from build123d import *

# Parameters (mm, degrees)
EXTRUDE_1_DEPTH        = 3
SKETCH_2_R             = 1.5
SKETCH_2_R_2           = 13.5
CUT_EXTRUDE_1333_DEPTH = 144.209636547
SKETCH_3_OUTSIDE_W     = 225.27
SKETCH_3_OUTSIDE_H     = 165.27
CUT_EXTRUDE_1_DEPTH    = 144.209636547
SKETCH_5_R             = 1.5
SKETCH_5_R_2           = 2
CUT_EXTRUDE_3_DEPTH    = 121.819741764
SKETCH_4_W             = 7
SKETCH_4_H             = 16
CUT_EXTRUDE_2_DEPTH    = 121.819741764
FILLET_1_R             = 2


with BuildPart() as part:
    # 草图1 → 凸台-拉伸1 (new body)
    with BuildSketch(Plane(origin=(0, 0, 0), x_dir=(1, 0, 0), z_dir=(0, 1, 0))):
        Polygon((-30, 60), (30, 60), (30, 33), (130, 33), (130, -33), (30, -33), (30, -60), (-30, -60), (-30, -30), (-50, -30), (-50, 30), (-30, 30), align=None)
    extrude(amount=EXTRUDE_1_DEPTH)

    # 草图2 → Cut-Extrude 1333 (cut, through all)
    with BuildSketch(Plane(origin=(0, 3, 0), x_dir=(1, 0, 0), z_dir=(0, 1, 0))):
        with Locations(Location((-30, 13, 0), (0, 0, 270))):
            Circle(SKETCH_2_R)
        with Locations(Location((-30, -13, 0), (0, 0, 270))):
            Circle(SKETCH_2_R)
        with Locations(Location((17.5, 36.9, 0), (0, 0, 270))):
            Circle(SKETCH_2_R)
        with Locations(Location((12.374368671, 24.525631329, 0), (0, 0, 270))):
            Circle(SKETCH_2_R)
        with Locations(Location((0, 19.4, 0), (0, 0, 270))):
            Circle(SKETCH_2_R)
        with Locations(Location((-12.374368671, 24.525631329, 0), (0, 0, 270))):
            Circle(SKETCH_2_R)
        with Locations(Location((-17.5, 36.9, 0), (0, 0, 270))):
            Circle(SKETCH_2_R)
        with Locations(Location((-12.374368671, 49.274368671, 0), (0, 0, 270))):
            Circle(SKETCH_2_R)
        with Locations(Location((0, 54.4, 0), (0, 0, 270))):
            Circle(SKETCH_2_R)
        with Locations(Location((12.374368671, 49.274368671, 0), (0, 0, 270))):
            Circle(SKETCH_2_R)
        with Locations(Location((12.374368671, -49.274368671, 0), (0, 0, 90))):
            Circle(SKETCH_2_R)
        with Locations(Location((0, -54.4, 0), (0, 0, 90))):
            Circle(SKETCH_2_R)
        with Locations(Location((-12.374368671, -49.274368671, 0), (0, 0, 90))):
            Circle(SKETCH_2_R)
        with Locations(Location((-17.5, -36.9, 0), (0, 0, 90))):
            Circle(SKETCH_2_R)
        with Locations(Location((-12.374368671, -24.525631329, 0), (0, 0, 90))):
            Circle(SKETCH_2_R)
        with Locations(Location((0, -19.4, 0), (0, 0, 90))):
            Circle(SKETCH_2_R)
        with Locations(Location((12.374368671, -24.525631329, 0), (0, 0, 90))):
            Circle(SKETCH_2_R)
        with Locations(Location((17.5, -36.9, 0), (0, 0, 90))):
            Circle(SKETCH_2_R)
        with Locations(Location((30, 13, 0), (0, 0, 270))):
            Circle(SKETCH_2_R)
        with Locations(Location((40, 13, 0), (0, 0, 270))):
            Circle(SKETCH_2_R)
        with Locations(Location((0, 36.9, 0), (0, 0, 270))):
            Circle(SKETCH_2_R_2)
        with Locations(Location((0, -36.9, 0), (0, 0, 90))):
            Circle(SKETCH_2_R_2)
        with Locations(Location((40, -13, 0), (0, 0, 90))):
            Circle(SKETCH_2_R)
        with Locations(Location((30, -13, 0), (0, 0, 90))):
            Circle(SKETCH_2_R)
        with Locations(Location((-30, 21.5, 0), (0, 0, 270))):
            Circle(SKETCH_2_R)
        with Locations(Location((-30, -21.5, 0), (0, 0, 90))):
            Circle(SKETCH_2_R)
    extrude(amount=-CUT_EXTRUDE_1333_DEPTH, mode=Mode.SUBTRACT)

    # 草图3 outside → 切除-拉伸1 (cut, through all)
    with BuildSketch(Plane(origin=(0, 0, 0), x_dir=(1, 0, 0), z_dir=(0, 1, 0))):
        with Locations((40, 0)):
            Rectangle(SKETCH_3_OUTSIDE_W, SKETCH_3_OUTSIDE_H)
        with BuildLine():
            Line((-21, 36.9), (-21, 26.5))
            Line((-21, 26.5), (-34, 26.5))
            Line((-34, 26.5), (-34, -26.5))
            Line((-34, -26.5), (-21, -26.5))
            Line((-21, -26.5), (-21, -36.9))
            ThreePointArc((-21, -36.9), (0, -57.9), (21, -36.9))
            Line((21, -36.9), (21, -33))
            Line((21, -33), (106, -33))
            Line((106, -33), (106, 33))
            Line((106, 33), (21, 33))
            Line((21, 33), (21, 36.9))
            ThreePointArc((21, 36.9), (0, 57.9), (-21, 36.9))
        make_face(mode=Mode.SUBTRACT)
    extrude(amount=CUT_EXTRUDE_1_DEPTH, mode=Mode.SUBTRACT)

    # 草图5 → 切除-拉伸3 (cut, through all)
    with BuildSketch(Plane(origin=(0, 3, 0), x_dir=(1, 0, 0), z_dir=(0, 1, 0))):
        with Locations(Location((81, 4, 0), (0, 0, 270))):
            Circle(SKETCH_5_R)
        with Locations(Location((101, 4, 0), (0, 0, 270))):
            Circle(SKETCH_5_R)
        with Locations(Location((101, -4, 0), (0, 0, 90))):
            Circle(SKETCH_5_R)
        with Locations(Location((81, -4, 0), (0, 0, 90))):
            Circle(SKETCH_5_R)
        with Locations(Location((69.5, 21.8, 0), (0, 0, 270))):
            Circle(SKETCH_5_R_2)
        with Locations(Location((85.5, 21.8, 0), (0, 0, 270))):
            Circle(SKETCH_5_R_2)
        with Locations(Location((49.5, -28.7, 0), (0, 0, 270))):
            Circle(SKETCH_5_R_2)
        with Locations(Location((89.5, -28.7, 0), (0, 0, 270))):
            Circle(SKETCH_5_R_2)
    extrude(amount=-CUT_EXTRUDE_3_DEPTH, mode=Mode.SUBTRACT)

    # 草图4 → 切除-拉伸2 (cut, through all)
    with BuildSketch(Plane(origin=(0, 3, 0), x_dir=(1, 0, 0), z_dir=(0, 1, 0))):
        Polygon((-15, -20.201242434), (-15, 20.201242434), (-3, 15.230679686), (-3, -15.230679686), align=None)
        with Locations((-30.5, 0)):
            Rectangle(SKETCH_4_W, SKETCH_4_H)
        Polygon((3, 15.230679686), (3, -15.230679686), (15, -20.201242434), (15, 20.201242434), align=None)
        Polygon((21, 33), (26, 28), (36, 28), (41, 33), align=None)
        Polygon((26, -8), (44, -8), (44, 8), (26, 8), (21, 8), (21, -8), align=None)
        Polygon((36, -28), (41, -33), (21, -33), (26, -28), align=None)
        with BuildLine():
            Line((53.5, 15), (68.5, 15))
            ThreePointArc((68.5, 15), (71.5, 12), (68.5, 9))
            Line((68.5, 9), (53.5, 9))
            ThreePointArc((53.5, 9), (50.5, 12), (53.5, 15))
        make_face()
        with BuildLine():
            Line((53.5, 3), (68.5, 3))
            ThreePointArc((68.5, 3), (71.5, 0), (68.5, -3))
            Line((68.5, -3), (53.5, -3))
            ThreePointArc((53.5, -3), (50.5, 0), (53.5, 3))
        make_face()
        with BuildLine():
            Line((53.5, -9), (68.5, -9))
            ThreePointArc((68.5, -9), (71.5, -12), (68.5, -15))
            Line((68.5, -15), (53.5, -15))
            ThreePointArc((53.5, -15), (50.5, -12), (53.5, -9))
        make_face()
    extrude(amount=-CUT_EXTRUDE_2_DEPTH, mode=Mode.SUBTRACT)

    # 圆角1
    fillet_1_edges = [part.edges().sort_by_distance(p)[0] for p in [
        (-21, 1.5, -26.5),
        (-34, 1.5, -26.5),
        (-34, 1.5, 26.5),
        (-21, 1.5, 26.5),
        (21, 1.5, 33),
        (106, 1.5, 33),
        (106, 1.5, -33),
        (21, 1.5, -33),
        (41, 1.5, -33),
        (36, 1.5, -28),
        (26, 1.5, -28),
        (26, 1.5, 28),
        (36, 1.5, 28),
        (41, 1.5, 33),
        (44, 1.5, -8),
        (44, 1.5, 8),
        (21, 1.5, 8),
        (21, 1.5, -8),
        (3, 1.5, -15.230679686),
        (15, 1.5, -20.201242434),
        (15, 1.5, 20.201242434),
        (3, 1.5, 15.230679686),
        (-27, 1.5, -8),
        (-27, 1.5, 8),
        (-34, 1.5, 8),
        (-34, 1.5, -8),
        (-15, 1.5, -20.201242434),
        (-3, 1.5, -15.230679686),
        (-3, 1.5, 15.230679686),
        (-15, 1.5, 20.201242434),
    ]]
    fillet(fillet_1_edges, radius=FILLET_1_R)


solid = part.part
The listing builds one solid part. Answer for the finished solid, in the listing's coordinates (mm). A direction names the side the tool comes from. Coordinates: 2 decimals unless noted, no trailing zeros. Loops run counter-clockwise (first coordinate to the right, second up) from the corner with the lowest first, then second, coordinate; pieces in that order, holes last.
1) Flat-ended cylindrical pins translate along their axes: pin 1 Ø3.5 at (x, z) = (0, 54.4) entering from +Y; pin 2 Ø0.9 at (x, y) = (64, 2) entering from +Z; pin 3 Ø1.5 at (x, y) = (58.5, 1.5) entering from -Z; pin 4 Ø1.5 at (y, z) = (2, 1) entering from -X. Find the tip coordinate at first contact, or state that the pin passes through.
2) Find the intervals of material crossed by L1, parallel to X at y = 0.8, z = -37; L2, parallel to Z at x = 81, y = 1.1; L3, parallel to Z at x = 34, y = 1.55, in increasing order.
3) Determine the mould class of faces 1 (the face through (-0.462, 1.479, 57.895)), 2 (the face through (-27, 1, -26.5)), 3 (the face through (-28.513, 1.521, 12.805)) for opening direction X: pulls with the +X half, pulls with the -X half, needs draft (parallel to the pull), parting line crosses it, or undercut.
4) A tool of negligible diameter and unlimited length cuts with its end or side. For faces 4 (the face through (21, 1, -35)), 5 (the face through (37, 0, 12)), 6 (the face through (38, 2, 30)), 7 (the face through (50.5, 1.5, 12.1)), 8 (the face through (31, 2, -28)), from which of +Z, -Z, +X, -X, +Y, -Y can it reach the whole face along a straight path? Write none if from no direction.
5) Find section A-A on x = 59.5. Write down the section's boundary in (y, z), then the cut area to 3 significant figures.
6) Find section B-B on z = 0. Write down the section's boundary in (x, y).
7) Find section C-C on x = 101. Write down the section's boundary in (y, z).
8) Find section D-D on z = 46. Write down the section's boundary in (x, y).
Values:
1. pin 1: stops at y = 3
1. pin 2: stops at z = 33
1. pin 3: stops at z = -33
1. pin 4: stops at x = -27
2. L1: x = -21 to -19, -16 to -13.5, 13.5 to 16, 19 to 21
2. L2: z = -33 to -5.5, -2.5 to 2.5, 5.5 to 33
2. L3: z = -28 to -8, 8 to 28
3. face 1: parting line crosses it
3. face 2: needs draft
3. face 3: undercut
4. face 4: -Z, +X, +Y, -Y
4. face 5: +Z, -Z, +X, -X, -Y
4. face 6: +Z, +Y, -Y
4. face 7: +Y, -Y
4. face 8: -Z, +Y, -Y
5. outline: (0, -33) - (3, -33) - (3, -15) - (0, -15) - close; (0, -9) - (3, -9) - (3, -3) - (0, -3) - close; (0, 3) - (3, 3) - (3, 9) - (0, 9) - close; (0, 15) - (3, 15) - (3, 33) - (0, 33) - close
5. area: 144 mm2
6. outline: (-27, 0) - (-15, 0) - (-15, 3) - (-27, 3) - close; (-3, 0) - (3, 0) - (3, 3) - (-3, 3) - close; (15, 0) - (21, 0) - (21, 3) - (15, 3) - close; (44, 0) - (50.5, 0) - (50.5, 3) - (44, 3) - close; (71.5, 0) - (106, 0) - (106, 3) - (71.5, 3) - close
7. outline: (0, -33) - (3, -33) - (3, -5.5) - (0, -5.5) - close; (0, -2.5) - (3, -2.5) - (3, 2.5) - (0, 2.5) - close; (0, 5.5) - (3, 5.5) - (3, 33) - (0, 33) - close
8. outline: (-18.93, 0) - (-9.97, 0) - (-9.97, 3) - (-18.93, 3) - close; (9.97, 0) - (18.93, 0) - (18.93, 3) - (9.97, 3) - close
